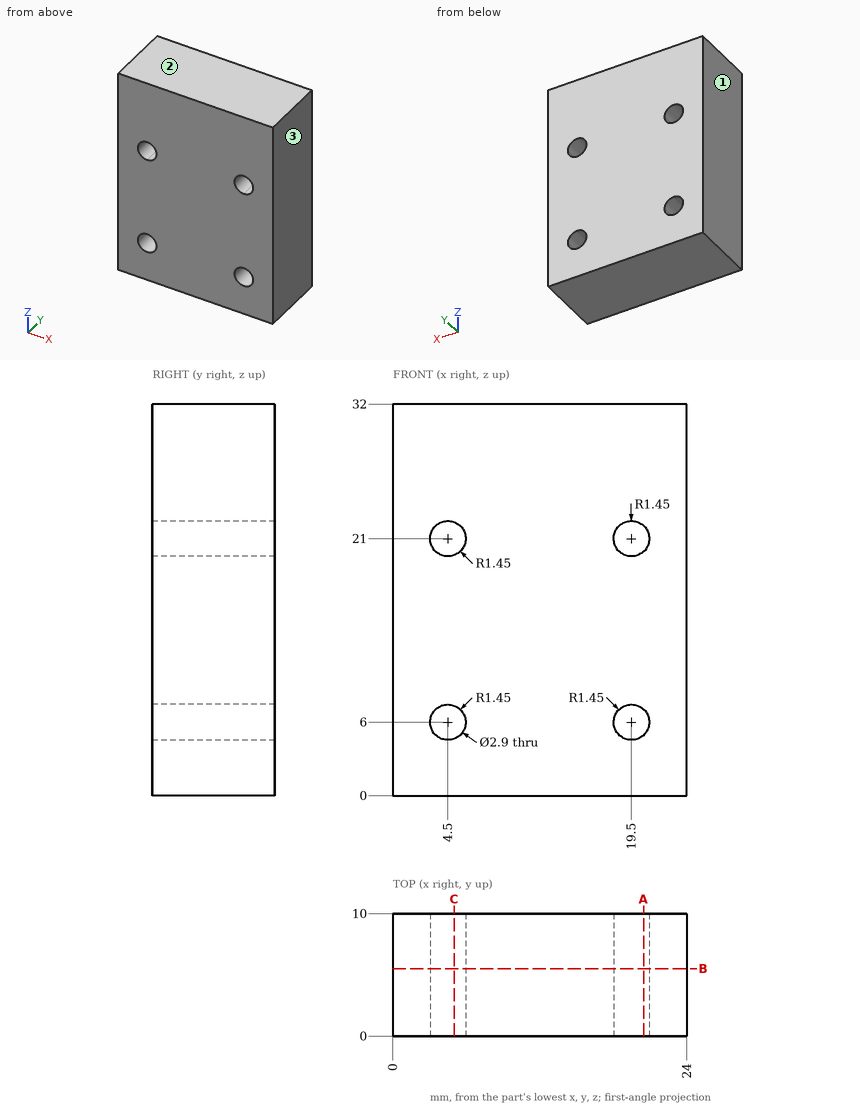
For this review, use the dimensioned drawing (mm, ordinates from the lowest corner) and the shaded views. Round coordinates to 2 decimals unless told otherwise and drop trailing zeros. Order: outer loops, then holes, each group sorted by start corner. A loop starts at its lowest first (then second) coordinate and runs counter-clockwise, first axis right, second up. Notation, with made-up numbers: (-12.5, -3) -> (13.5, -3) arc R21 cw to (13.5, 35) -> close; hole circle Ø8 at (57.5, 57). An arc over 180 degrees is marked (long way). One line per item, written item: value. Start each with the question number.
Q1. Take a section at B-B (y = 5.5). Write out the cut boundary in (x, z).
Q2. Wall thickness on line 1 (Z direction, x = 4.5, y = 7.75); line 2 (X direction, y = 4.5, z = 7); line 3 (Z direction, x = 18.75, y = 8): over which ranges is each line inside the solid? List them lowest first.
Q3. Take a section at C-C (x = 5). Write out the cut boundary in (y, z).
Q4. Take a section at A-A (x = 20.5). Write out the cut boundary in (y, z).
Q5. Mouldability with a two-part tool opening along X and no side actions: class the marked faces 1, 2 and 3 as released by +X, released by -X, zero draft, split by the parting line, or undercut.
Reported:
1. outline: (0, 0) -> (24, 0) -> (24, 32) -> (0, 32) -> close; hole circle Ø2.9 at (4.5, 6); hole circle Ø2.9 at (4.5, 21); hole circle Ø2.9 at (19.5, 6); hole circle Ø2.9 at (19.5, 21)
2. line 1: z = 0 to 4.55, 7.45 to 19.55, 22.45 to 32
2. line 2: x = 0 to 3.45, 5.55 to 18.45, 20.55 to 24
2. line 3: z = 0 to 4.76, 7.24 to 19.76, 22.24 to 32
3. outline: (0, 0) -> (10, 0) -> (10, 4.64) -> (0, 4.64) -> close; (0, 7.36) -> (10, 7.36) -> (10, 19.64) -> (0, 19.64) -> close; (0, 22.36) -> (10, 22.36) -> (10, 32) -> (0, 32) -> close
4. outline: (0, 0) -> (10, 0) -> (10, 4.95) -> (0, 4.95) -> close; (0, 7.05) -> (10, 7.05) -> (10, 19.95) -> (0, 19.95) -> close; (0, 22.05) -> (10, 22.05) -> (10, 32) -> (0, 32) -> close
5. face 1: released by -X
5. face 2: zero draft
5. face 3: released by +X
